Part print with two shaded views. Sizes in mm from the minimum x, y, z corner. A direction names the side the tool comes from. Round coordinates to 2 decimals unless told otherwise and drop trailing zeros. Order: outer loops, then holes, each group sorted by start corner. A loop starts at its lowest first (then second) coordinate and runs counter-clockwise, first axis right, second up. Notation, with made-up numbers: (52.5, 57.25) -> (78.5, 57.25) arc R17 ccw to (78.5, 68.25) -> close; hole circle Ø1 at (41.25, -15). An arc over 180 degrees is marked (long way). Put each result on its own line as item: value. Start each with the question number.
Q1. Pull direction Y, two halves, no side cores. Call the marked faces 3, 4 and 5: released by +Y, released by -Y, zero draft, split by the parting line, or undercut.
Q2. Cut at B-B, the plane x = 5.5. List the corners of the cut face in (y, z).
Q3. 3-axis set-ups, long thin cutter, end or side, ignore diameter. For the marked faces 1 and 2: which of +Z, -Z, +X, -X, +Y, -Y reach the whole face in a straight line?
Q4. Cut at C-C, the plane z = 3. List the corners of the cut face in (x, y).
Q5. Cut at D-D, the plane x = 2.5. List the corners of the cut face in (y, z).
Q6. Cut at A-A, the plane y = 3. List the corners of the cut face in (x, z).
Q7. Flat gauge pins, fed straight in: P1, Ø0.8, axis at x = 5.5, z = 1, coming from the +Y side; P2, Ø0.8, axis at y = 3, z = 4.5, coming from the +X side; P3, Ø0.5, axis at x = 5.5, z = 1, coming from the -Y side. Where does each tip first touch, or does it go through?
Q8. Probe L1, parallel to Y at x = 4.4, z = 3; L2, parallel to Z at x = 4.4, y = 2.5; L3, parallel to Y at x = 1.95, z = 3.75. List the from-to ranges inside material, lowest first.
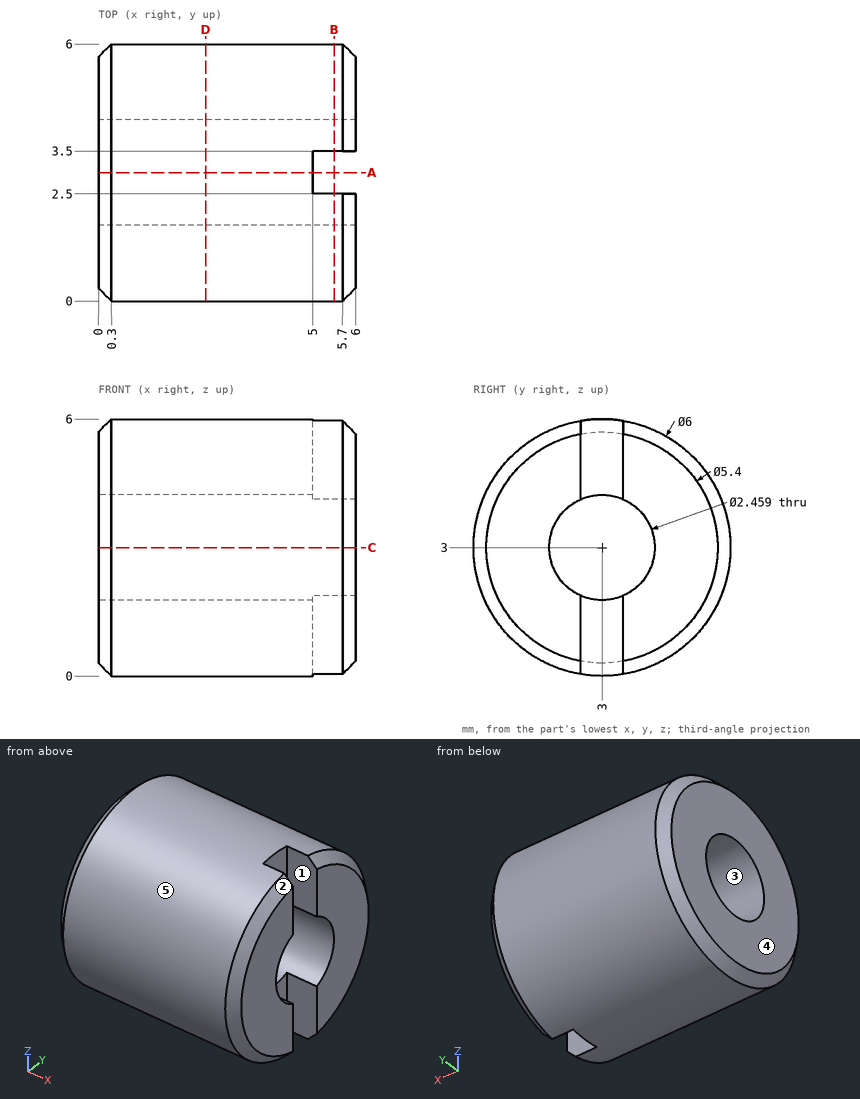
Ans:
1. face 3: undercut
1. face 4: zero draft
1. face 5: split by the parting line
2. outline: (2.5, 0.04) -> (2.5, 1.88) arc R1.23 cw to (2.5, 4.12) -> (2.5, 5.96) arc R3 ccw to start; (3.5, 0.04) arc R3 ccw to (3.5, 5.96) -> (3.5, 4.12) arc R1.23 cw to (3.5, 1.88) -> close
3. face 1: +Z, -Z, +X
3. face 2: +X, -Y
4. outline: (0, 0.3) -> (0.3, 0) -> (5.7, 0) -> (6, 0.3) -> (6, 1.77) -> (0, 1.77) -> close; (0, 4.23) -> (6, 4.23) -> (6, 5.7) -> (5.7, 6) -> (0.3, 6) -> (0, 5.7) -> close
5. outline: circle Ø6 at (3, 3); hole circle Ø2.46 at (3, 3)
6. outline: (0, 0.3) -> (0.3, 0) -> (5, 0) -> (5, 1.77) -> (0, 1.77) -> close; (0, 4.23) -> (5, 4.23) -> (5, 6) -> (0.3, 6) -> (0, 5.7) -> close
7. P1: stops at y = 5.54
7. P2: stops at x = 5
7. P3: stops at y = 0.56
8. L1: y = 0 to 1.77, 4.23 to 6
8. L2: z = 0.04 to 1.88, 4.12 to 5.96
8. L3: y = 0.1 to 2.03, 3.97 to 5.9
